Build history of the part. All positions in model axes, mm. A direction names the side the tool comes from. Give positions to 0.01 mm unless a question says otherwise; leave off trailing zeros. Order: outer loops, then holes, each group sorted by start corner. A loop starts at its lowest first (then second) coordinate and runs counter-clockwise, first axis right, second up. Notation, with made-up numbers: (30.5, 74) - (82.5, 74) arc R18 ccw to (82.5, 107) - close; hole circle Ø2 at (-36.5, 19). An arc over 180 degrees is marked (long way). Use a Markdown table: item, result.
from build123d import *

# Parameters (mm, degrees)
BOSS_EXTRUDE1_DEPTH = 63.5
SKETCH3_W           = 381
SKETCH3_H           = 9.525
CUT_EXTRUDE1_DEPTH  = 63.5
SKETCH4_W           = 381
SKETCH4_H           = 9.525
CUT_EXTRUDE2_DEPTH  = 63.5
CUT_EXTRUDE3_DEPTH  = 31.75
CUT_EXTRUDE4_DEPTH  = 76.2
CUT_EXTRUDE5_DEPTH  = 57.15
CUT_EXTRUDE6_DEPTH  = 31.75
CUT_EXTRUDE7_DEPTH  = 76.2
CUT_EXTRUDE8_DEPTH  = 57.15
FILLET1_R           = 5.08
SKETCH12_W          = 50.8
SKETCH12_H          = 38.1
BOSS_EXTRUDE2_DEPTH = 1.5875
SKETCH13_R          = 11.1125
SKETCH13_R_2        = 9.525
BOSS_EXTRUDE3_DEPTH = 12.7
BOSS_EXTRUDE4_START = -6.35
SKETCH15_R          = 9.525
BOSS_EXTRUDE4_DEPTH = 6.35
SKETCH16_R          = 0.79375
BOSS_EXTRUDE5_DEPTH = 11.43
FILLET2_R           = 0.79375
SKETCH17_R          = 3.175
CUT_EXTRUDE9_DEPTH  = 25.4


with BuildPart() as part:
    # Sketch1 → Boss-Extrude1 (new body)
    with BuildSketch(Plane(origin=(0, 0, 0), x_dir=(1, 0, 0), z_dir=(0, 1, 0))):
        Polygon((-146.05, 190.5), (-190.5, 146.05), (-190.5, -146.05), (-146.05, -190.5), (146.05, -190.5), (190.5, -146.05), (190.5, 146.05), (146.05, 190.5), align=None)
    extrude(amount=BOSS_EXTRUDE1_DEPTH)

    # Sketch3 → Cut-Extrude1 (cut)
    with BuildSketch(Plane.XY.offset(190.5)):
        with Locations((0, 31.75)):
            Rectangle(SKETCH3_W, SKETCH3_H)
    cut_extrude1 = extrude(amount=-CUT_EXTRUDE1_DEPTH, mode=Mode.SUBTRACT)

    # Mirror1: Cut-Extrude1 across plane
    add(cut_extrude1.mirror(Plane.XY), mode=Mode.SUBTRACT)

    # Sketch4 → Cut-Extrude2 (cut)
    with BuildSketch(Plane.ZY.offset(190.5)):
        with Locations((0, 31.75)):
            Rectangle(SKETCH4_W, SKETCH4_H)
    cut_extrude2 = extrude(amount=-CUT_EXTRUDE2_DEPTH, mode=Mode.SUBTRACT)

    # Mirror2: Cut-Extrude2 across plane
    add(cut_extrude2.mirror(Plane(origin=(0, 0, 0), x_dir=(0, 0, 1), z_dir=(1, 0, 0))), mode=Mode.SUBTRACT)

    # Sketch5 → Cut-Extrude3 (cut)
    with BuildSketch(Plane(origin=(0, 63.5, 0), x_dir=(1, 0, 0), z_dir=(0, 1, 0))):
        with BuildLine():
            Line((31.75, -179.3875), (-31.75, -179.3875))
            ThreePointArc((-31.75, -179.3875), (-44.45, -166.6875), (-31.75, -153.9875))
            Line((-31.75, -153.9875), (31.75, -153.9875))
            ThreePointArc((31.75, -153.9875), (44.45, -166.6875), (31.75, -179.3875))
        make_face()
    extrude(amount=-CUT_EXTRUDE3_DEPTH, mode=Mode.SUBTRACT)

    # Sketch6 → Cut-Extrude4 (cut)
    with BuildSketch(Plane.XY.offset(190.5)):
        with BuildLine():
            Line((-38.1, 26.9875), (38.1, 26.9875))
            Line((38.1, 26.9875), (38.1, 10.583333333))
            ThreePointArc((38.1, 10.583333333), (36.860085374, 7.589914626), (33.866666667, 6.35))
            Line((33.866666667, 6.35), (-33.866666667, 6.35))
            ThreePointArc((-33.866666667, 6.35), (-36.860085374, 7.589914626), (-38.1, 10.583333333))
            Line((-38.1, 10.583333333), (-38.1, 26.9875))
        make_face()
        with BuildLine():
            Line((-12.7, 36.5125), (12.7, 36.5125))
            Line((12.7, 36.5125), (12.7, 40.3225))
            ThreePointArc((12.7, 40.3225), (11.956051224, 42.118551224), (10.16, 42.8625))
            Line((10.16, 42.8625), (-10.16, 42.8625))
            ThreePointArc((-10.16, 42.8625), (-11.956051224, 42.118551224), (-12.7, 40.3225))
            Line((-12.7, 40.3225), (-12.7, 36.5125))
        make_face()
    extrude(amount=-CUT_EXTRUDE4_DEPTH, mode=Mode.SUBTRACT)

    # Sketch7 → Cut-Extrude5 (cut)
    with BuildSketch(Plane.XY.offset(166.6875)):
        with BuildLine():
            Line((-38.1, 26.9875), (-38.1, 10.583333333))
            ThreePointArc((-38.1, 10.583333333), (-36.860085374, 7.589914626), (-33.866666667, 6.35))
            Line((-33.866666667, 6.35), (33.866666667, 6.35))
            ThreePointArc((33.866666667, 6.35), (36.860085374, 7.589914626), (38.1, 10.583333333))
            Line((38.1, 10.583333333), (38.1, 26.9875))
            Line((38.1, 26.9875), (-38.1, 26.9875))
        make_face()
        Polygon((44.45, 26.9875), (38.1, 26.9875), (-38.1, 26.9875), (-44.45, 26.9875), (-44.45, 60.325), (44.45, 60.325), align=None)
    extrude(amount=-CUT_EXTRUDE5_DEPTH, mode=Mode.SUBTRACT)

    # Sketch8 → Cut-Extrude6 (cut)
    with BuildSketch(Plane.XZ):
        with BuildLine():
            Line((31.75, -179.3875), (-31.75, -179.3875))
            ThreePointArc((-31.75, -179.3875), (-44.45, -166.6875), (-31.75, -153.9875))
            Line((-31.75, -153.9875), (31.75, -153.9875))
            ThreePointArc((31.75, -153.9875), (44.45, -166.6875), (31.75, -179.3875))
        make_face()
    extrude(amount=-CUT_EXTRUDE6_DEPTH, mode=Mode.SUBTRACT)

    # Sketch9 → Cut-Extrude7 (cut)
    with BuildSketch(Plane(origin=(0, 0, -190.5), x_dir=(-1, 0, 0), z_dir=(0, 0, -1))):
        with BuildLine():
            Line((33.866666667, 57.15), (-33.866666667, 57.15))
            ThreePointArc((-33.866666667, 57.15), (-36.860085374, 55.910085374), (-38.1, 52.916666667))
            Line((-38.1, 52.916666667), (-38.1, 36.5125))
            Line((-38.1, 36.5125), (38.1, 36.5125))
            Line((38.1, 36.5125), (38.1, 52.916666667))
            ThreePointArc((38.1, 52.916666667), (36.860085374, 55.910085374), (33.866666667, 57.15))
        make_face()
        with BuildLine():
            Line((10.16, 20.6375), (-10.16, 20.6375))
            ThreePointArc((-10.16, 20.6375), (-11.956051224, 21.381448776), (-12.7, 23.1775))
            Line((-12.7, 23.1775), (-12.7, 26.9875))
            Line((-12.7, 26.9875), (12.7, 26.9875))
            Line((12.7, 26.9875), (12.7, 23.1775))
            ThreePointArc((12.7, 23.1775), (11.956051224, 21.381448776), (10.16, 20.6375))
        make_face()
    extrude(amount=-CUT_EXTRUDE7_DEPTH, mode=Mode.SUBTRACT)

    # Sketch10 → Cut-Extrude8 (cut)
    with BuildSketch(Plane(origin=(0, 0, -166.6875), x_dir=(-1, 0, 0), z_dir=(0, 0, -1))):
        Polygon((-44.45, 36.5125), (-38.1, 36.5125), (38.1, 36.5125), (44.45, 36.5125), (44.45, 3.175), (-44.45, 3.175), align=None)
        with BuildLine():
            Line((38.1, 36.5125), (38.1, 52.916666667))
            ThreePointArc((38.1, 52.916666667), (36.860085374, 55.910085374), (33.866666667, 57.15))
            Line((33.866666667, 57.15), (-33.866666667, 57.15))
            ThreePointArc((-33.866666667, 57.15), (-36.860085374, 55.910085374), (-38.1, 52.916666667))
            Line((-38.1, 52.916666667), (-38.1, 36.5125))
            Line((-38.1, 36.5125), (38.1, 36.5125))
        make_face()
    extrude(amount=-CUT_EXTRUDE8_DEPTH, mode=Mode.SUBTRACT)

    # Fillet1
    fillet1_edges = [part.edges().sort_by_distance(p)[0] for p in [
        (-190.5, 63.5, 0),
        (-168.275, 0, -168.275),
        (0, 0, -190.5),
        (-168.275, 63.5, 168.275),
        (0, 63.5, 190.5),
        (168.275, 63.5, 168.275),
        (190.5, 63.5, 0),
        (168.275, 63.5, -168.275),
        (0, 63.5, -190.5),
        (-168.275, 63.5, -168.275),
        (168.275, 0, -168.275),
        (190.5, 0, 0),
        (168.275, 0, 168.275),
        (0, 0, 190.5),
        (-168.275, 0, 168.275),
        (-190.5, 0, 0),
    ]]
    fillet(fillet1_edges, radius=FILLET1_R)

    # Sketch12 → Boss-Extrude2 (add)
    with BuildSketch(Plane.XY.offset(152.4)):
        with Locations((0, 25.4)):
            Rectangle(SKETCH12_W, SKETCH12_H)
    extrude(amount=-BOSS_EXTRUDE2_DEPTH)

    # Sketch13 → Boss-Extrude3 (add)
    with BuildSketch(Plane.XY.offset(152.4)):
        with Locations(Location((0, 25.4, 0), (0, 0, 180))):
            Circle(SKETCH13_R)
        with Locations((0, 25.4)):
            Circle(SKETCH13_R_2, mode=Mode.SUBTRACT)
    extrude(amount=BOSS_EXTRUDE3_DEPTH)

    # Sketch15 → Boss-Extrude4 (add)
    with BuildSketch(Plane.XY.offset(152.4).offset(BOSS_EXTRUDE4_START)):
        with Locations((0, 25.4)):
            Circle(SKETCH15_R)
    extrude(amount=BOSS_EXTRUDE4_DEPTH)

    # Sketch16 → Boss-Extrude5 (add)
    with BuildSketch(Plane.XY.offset(152.4)):
        with Locations(Location((2.694076836, 28.094076836, 0), (0, 0, 180))):
            Circle(SKETCH16_R)
        with Locations(Location((-2.694076836, 28.094076836, 0), (0, 0, 180))):
            Circle(SKETCH16_R)
        with Locations(Location((-2.694076836, 22.705923164, 0), (0, 0, 180))):
            Circle(SKETCH16_R)
        with Locations(Location((2.694076836, 22.705923164, 0), (0, 0, 180))):
            Circle(SKETCH16_R)
    extrude(amount=BOSS_EXTRUDE5_DEPTH)

    # Fillet2
    fillet2_edges = [part.edges().sort_by_distance(p)[0] for p in [
        (3.487826836, 28.094076836, 163.83),
        (-1.900326836, 28.094076836, 163.83),
        (-1.900326836, 22.705923164, 163.83),
        (3.487826836, 22.705923164, 163.83),
    ]]
    fillet(fillet2_edges, radius=FILLET2_R)

    # Sketch17 → Cut-Extrude9 (cut)
    with BuildSketch(Plane.XZ):
        with Locations(Location((165.1, 0, 0), (0, 0, 270))):
            Circle(SKETCH17_R)
        with Locations(Location((-165.1, 0, 0), (0, 0, 90))):
            Circle(SKETCH17_R)
    extrude(amount=-CUT_EXTRUDE9_DEPTH, mode=Mode.SUBTRACT)


solid = part.part
1) Two-plate mould, pull along Z, no slides. Class faces 4 (the flat face through (0, 26, 146.05)), 5 (the flat face through (168.59, 15.88, -167.96)), 6 (the flat face through (140, 36.512, -3)): +Z half, -Z half, draft (parallel to the pull), parting line (faces both ways), or undercut.
Computed:
| item | result |
|---|---|
| face 4 | undercut |
| face 5 | -Z half |
| face 6 | draft |
2) Slice it at B-B (x = 120). Write the cut outline in (y, z), and give its area (3 significant figures).
Computed:
| item | result |
|---|---|
| outline | (0, -185.42) arc R5.08 ccw to (5.08, -190.5) - (26.99, -190.5) - (26.99, -127) - (36.51, -127) - (36.51, -190.5) - (58.42, -190.5) arc R5.08 ccw to (63.5, -185.42) - (63.5, 185.42) arc R5.08 ccw to (58.42, 190.5) - (36.51, 190.5) - (36.51, 127) - (26.99, 127) - (26.99, 190.5) - (5.08, 190.5) arc R5.08 ccw to (0, 185.42) - close |
| area | 23,000 mm² |
3) Pin check, flat tips, straight feed: P1, Ø3.5, axis at x = -7, y = 1.5, coming from the -Z side; P2, Ø3, axis at x = 72.5, y = 31.5, coming from the +Z side; P3, Ø3, axis at x = 164, z = 0, coming from the -Y side. Stop position of each tip, or through.
Computed:
| item | result |
|---|---|
| P1 | stops at z = -190.16 |
| P2 | stops at z = 127 |
| P3 | stops at y = 25.4 |
4) Slice it at A-A (z = 28.5). Write the cut outline in (x, y), and give its area (3 significant figures).
Computed:
| item | result |
|---|---|
| outline | (-190.5, 5.08) arc R5.08 ccw to (-185.42, 0) - (185.42, 0) arc R5.08 ccw to (190.5, 5.08) - (190.5, 26.99) - (127, 26.99) - (127, 36.51) - (190.5, 36.51) - (190.5, 58.42) arc R5.08 ccw to (185.42, 63.5) - (-185.42, 63.5) arc R5.08 ccw to (-190.5, 58.42) - (-190.5, 36.51) - (-127, 36.51) - (-127, 26.99) - (-190.5, 26.99) - close |
| area | 23,000 mm² |
5) Wall check: line 1 (X direction, y = 11.25, z = 0) (3 decimals); line 2 (X direction, y = 54, z = 140.5); line 3 (Z direction, x = 12, y = 32.5). Give the ranges that are in metal, low to high. Write a range as from..to.
Computed:
| item | result |
|---|---|
| line 1 | x = -190.5..-168.275, -161.925..161.925, 168.275..190.5 |
| line 2 | x = -190.5..-44.45, 44.45..190.5 |
| line 3 | z = -109.54..109.54, 150.81..152.4 |
6) Tool access for faces 1 (the cylindrical face through (-41.3, 13.3, -175.06)), 2 (the flat face through (-86, 32, -127)), 3 (the flat face through (-86, 32, 127)): list every direction of +Z, -Z, +X, -X, +Y, -Y with a clear straight run to the whole face (end or side of a thin tool).
Computed:
| item | result |
|---|---|
| face 1 | -Y |
| face 2 | -Z, +X, -X |
| face 3 | +Z, +X, -X |
